from build123d import *

# Parameters (mm, degrees)
SKETCH1_W           = 42
SKETCH1_H           = 42
BOSS_EXTRUDE1_DEPTH = 37
FILLET1_R           = 5.5
SKETCH2_R           = 4
SKETCH2_R_2         = 3
CUT_EXTRUDE1_DEPTH  = 2
SKETCH4_R           = 2.5
BOSS_EXTRUDE2_DEPTH = 25
SKETCH5_R           = 1.5
CUT_EXTRUDE2_DEPTH  = 8
CUT_EXTRUDE3_START  = -12
SKETCH6_R           = 34.308404515
CUT_EXTRUDE3_DEPTH  = 12
CHAMFER1_SIZE       = 0.5
SKETCH7_R           = 11
BOSS_EXTRUDE3_DEPTH = 1


with BuildPart() as part:
    # Sketch1 → Boss-Extrude1 (new body)
    with BuildSketch(Plane.XY):
        Rectangle(SKETCH1_W, SKETCH1_H)
    extrude(amount=BOSS_EXTRUDE1_DEPTH)

    # Fillet1
    fillet1_edges = [part.edges().sort_by_distance(p)[0] for p in [
        (21, -21, 18.5),
        (-21, -21, 18.5),
        (-21, 21, 18.5),
        (21, 21, 18.5),
    ]]
    fillet(fillet1_edges, radius=FILLET1_R)

    # Sketch2 → Cut-Extrude1 (cut)
    with BuildSketch(Plane.XY.offset(37)):
        Circle(SKETCH2_R)
        with Locations((15.5, -15.5)):
            Circle(SKETCH2_R_2)
        with Locations((15.5, 15.5)):
            Circle(SKETCH2_R_2)
        with Locations((-15.5, 15.5)):
            Circle(SKETCH2_R_2)
        with Locations((-15.5, -15.5)):
            Circle(SKETCH2_R_2)
    extrude(amount=-CUT_EXTRUDE1_DEPTH, mode=Mode.SUBTRACT)

    # Sketch4 → Boss-Extrude2 (add)
    with BuildSketch(Plane(origin=(0, 0, 0), x_dir=(-1, 0, 0), z_dir=(0, 0, -1))):
        Circle(SKETCH4_R)
    extrude(amount=BOSS_EXTRUDE2_DEPTH)

    # Sketch5 → Cut-Extrude2 (cut)
    with BuildSketch(Plane(origin=(0, 0, 0), x_dir=(-1, 0, 0), z_dir=(0, 0, -1))):
        with Locations((15.5, -15.5)):
            Circle(SKETCH5_R)
        with Locations((-15.5, -15.5)):
            Circle(SKETCH5_R)
        with Locations((15.5, 15.5)):
            Circle(SKETCH5_R)
        with Locations((-15.5, 15.5)):
            Circle(SKETCH5_R)
    extrude(amount=-CUT_EXTRUDE2_DEPTH, mode=Mode.SUBTRACT)

    # Sketch6 → Cut-Extrude3 (cut)
    # profile 1 of 2: a face of its own
    with BuildSketch(Plane.XY.offset(37).offset(CUT_EXTRUDE3_START)):
        Circle(SKETCH6_R)
        with BuildLine():
            Line((-21, 15.5), (-21, -15.5))
            ThreePointArc((-21, -15.5), (-19.389087297, -19.389087297), (-15.5, -21))
            Line((-15.5, -21), (15.5, -21))
            ThreePointArc((15.5, -21), (19.389087297, -19.389087297), (21, -15.5))
            Line((21, -15.5), (21, 15.5))
            ThreePointArc((21, 15.5), (19.389087297, 19.389087297), (15.5, 21))
            Line((15.5, 21), (-15.5, 21))
            ThreePointArc((-15.5, 21), (-19.389087297, 19.389087297), (-21, 15.5))
        make_face(mode=Mode.SUBTRACT)
    # profile 2 of 2: a face of its own
    with BuildSketch(Plane.XY.offset(37).offset(CUT_EXTRUDE3_START)):
        with BuildLine():
            ThreePointArc((-15.5, 21), (-19.389087297, 19.389087297), (-21, 15.5))
            Line((-21, 15.5), (-21, -15.5))
            ThreePointArc((-21, -15.5), (-19.389087297, -19.389087297), (-15.5, -21))
            Line((-15.5, -21), (15.5, -21))
            ThreePointArc((15.5, -21), (19.389087297, -19.389087297), (21, -15.5))
            Line((21, -15.5), (21, 15.5))
            ThreePointArc((21, 15.5), (19.389087297, 19.389087297), (15.5, 21))
            Line((15.5, 21), (-15.5, 21))
        make_face()
        with BuildLine():
            ThreePointArc((-15.5, 20.5), (-19.035533906, 19.035533906), (-20.5, 15.5))
            Line((-20.5, 15.5), (-20.5, -15.5))
            ThreePointArc((-20.5, -15.5), (-19.035533906, -19.035533906), (-15.5, -20.5))
            Line((-15.5, -20.5), (15.5, -20.5))
            ThreePointArc((15.5, -20.5), (19.035533906, -19.035533906), (20.5, -15.5))
            Line((20.5, -15.5), (20.5, 15.5))
            ThreePointArc((20.5, 15.5), (19.035533906, 19.035533906), (15.5, 20.5))
            Line((15.5, 20.5), (-15.5, 20.5))
        make_face(mode=Mode.SUBTRACT)
    extrude(amount=-CUT_EXTRUDE3_DEPTH, mode=Mode.SUBTRACT)

    # Chamfer1
    chamfer1_edges = [part.edges().sort_by_distance(p)[0] for p in [
        (0, -21, 0),
        (0, -21, 37),
        (21, 0, 0),
        (-21, 0, 0),
        (0, 21, 0),
        (-19.389087297, 19.389087297, 0),
        (19.389087297, 19.389087297, 0),
        (19.389087297, -19.389087297, 0),
        (-19.389087297, -19.389087297, 0),
        (-21, 0, 37),
        (21, 0, 37),
        (0, 21, 37),
        (-19.389087297, 19.389087297, 37),
        (19.389087297, 19.389087297, 37),
        (19.389087297, -19.389087297, 37),
        (-19.389087297, -19.389087297, 37),
        (-4, 0, 37),
        (12.5, -15.5, 37),
        (12.5, 15.5, 37),
        (-18.5, 15.5, 37),
        (-18.5, -15.5, 37),
        (2.5, 0, 0),
        (2.5, 0, -25),
        (-14, -15.5, 0),
        (17, -15.5, 0),
        (-14, 15.5, 0),
        (17, 15.5, 0),
    ]]
    chamfer(chamfer1_edges, length=CHAMFER1_SIZE)

    # Sketch7 → Boss-Extrude3 (add)
    with BuildSketch(Plane(origin=(0, 0, 0), x_dir=(-1, 0, 0), z_dir=(0, 0, -1))):
        Circle(SKETCH7_R)
    extrude(amount=BOSS_EXTRUDE3_DEPTH)


solid = part.part
The listing builds one solid part. Answer for the finished solid, in the listing's coordinates (mm). A direction names the side the tool comes from. Coordinates: 2 decimals unless noted, no trailing zeros. Loops run counter-clockwise (first coordinate to the right, second up) from the corner with the lowest first, then second, coordinate; pieces in that order, holes last. Notation, with made-up numbers: (75, -8) -> (115, -8) arc R17 cw to (115, 6) -> close; hole circle Ø11 at (30.5, 87). An arc over 180 degrees is marked (long way). Answer in a Markdown table with one row per item. Add a question column.
1. Determine the mould class of faces 1 (the cylindrical face through (0.54, -2.44, -12.59)), 2 (the flat face through (0, -20.5, 19)), 3 (the flat face through (-20.5, 0, 19)), 4 (the cylindrical face through (-14, -15.43, 4.2)) for opening direction Y: +Y half, -Y half, draft (parallel to the pull), parting line (faces both ways), or undercut.
2. Flat-ended cylindrical pins translate along their axes: P1, Ø3, axis at x = -9, z = -2, coming from the +Y side; P2, Ø3, axis at x = -14.5, y = 15.5, coming from the +Z side; P3, Ø3, axis at x = 17, y = -15, coming from the +Z side. Find the tip coordinate at first contact, or state that the pin passes through.
3. The part is cut by section D-D, the plane z = 15.5. Write down the section's boundary in (x, y), then the cut area to 3 significant figures.
4. The part is cut by section A-A, the plane z = 4. Write down the section's boundary in (x, y).
5. Consider line 1 (Y direction, x = 15.5, z = 5); line 2 (Y direction, x = -15.5, z = 35.4); line 3 (X direction, y = -15, z = 6). Determine where each line is inside the solid, lowest interval first. Write a range as [from, to].
6. For faces 5 (the flat face through (0, 21, 7)), 6 (the flat face through (16, 16, 8)), 7 (the cylindrical face through (-19.07, -19, 19.08)), 8 (the flat face through (15, -15, 35)), determine the directions among +Z, -Z, +X, -X, +Y, -Y from which every point of the face is accessible in a straight line to the end or side of a thin tool.
Answer below:
| question | item | result |
|---|---|---|
| 1 | face 1 | parting line |
| 1 | face 2 | -Y half |
| 1 | face 3 | draft |
| 1 | face 4 | undercut |
| 2 | P1 | y = 7.67 |
| 2 | P2 | z = 35 |
| 2 | P3 | z = 36.58 |
| 3 | outline | (-20.5, -15.5) arc R5 ccw to (-15.5, -20.5) -> (15.5, -20.5) arc R5 ccw to (20.5, -15.5) -> (20.5, 15.5) arc R5 ccw to (15.5, 20.5) -> (-15.5, 20.5) arc R5 ccw to (-20.5, 15.5) -> close |
| 3 | area | 1,660 mm2 |
| 4 | outline | (-21, -15.5) arc R5.5 ccw to (-15.5, -21) -> (15.5, -21) arc R5.5 ccw to (21, -15.5) -> (21, 15.5) arc R5.5 ccw to (15.5, 21) -> (-15.5, 21) arc R5.5 ccw to (-21, 15.5) -> close; hole circle Ø3 at (-15.5, -15.5); hole circle Ø3 at (-15.5, 15.5); hole circle Ø3 at (15.5, -15.5); hole circle Ø3 at (15.5, 15.5) |
| 5 | line 1 | [-21, -17], [-14, 14], [17, 21] |
| 5 | line 2 | [-21, -18.5], [-12.5, 12.5], [18.5, 21] |
| 5 | line 3 | [-21, -16.91], [-14.09, 14.09], [16.91, 21] |
| 6 | face 5 | +Z, -Z, +X, -X, +Y |
| 6 | face 6 | -Z |
| 6 | face 7 | -X, -Y |
| 6 | face 8 | +Z |
